CAD build for the part. Positions are in the model's coordinates, mm. Coordinates: 2 decimals unless noted, no trailing zeros. Write each loop counter-clockwise with the first axis right and the second up, starting at its lowest first coordinate (ties: lowest second). Pieces come first, ordered by that corner, then holes. Notation, with made-up numbers: (30, -9) -> (74, -9) arc R16 cw to (74, 22) -> close; hole circle Ø9 at (20, -15). An arc over 180 degrees is marked (long way). Answer as CSV lines item,"result".
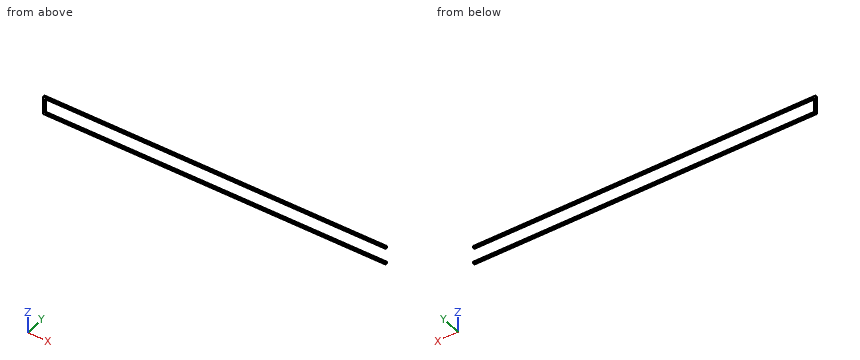
Autodesk Inventor part; units mm, degrees
ref_plane "Work Plane1" through (6.35, 0, 0) normal (1, 0, 0) x (0, 1, 0)
ref_plane "Work Plane2" through (0, 0, -6.35) normal (0, 0, 1) x (1, 0, 0)
ref_plane "XZ Plane" through (0, 0, 0) normal (0, 1, 0) x (-1, 0, 0)
sketch "Sketch1" plane through (0, 0, 0) normal (0, 1, 0) x (-1, 0, 0)
  line L0 (0, 0) -> (47.625, 0)
  line L1 (47.625, -2.54) -> (0, -2.54)
  line L2 (47.625, -2.54) -> (47.625, 0)
  dimension "d69" = 47.625
  dimension "d70" = 47.625
  dimension "d89" = 2.54
  dimension "d90" = 0
  dimension "d91" = 0
  dimension "d92" = 0
sketch "Sketch2" plane through (0, 0, 0) normal (1, 0, 0) x (0, 1, 0)
  line L0 (0, 0) -> (0.254, 0)
  line L1 (0.254, 0) -> (0.254, -0.254)
  line L2 (0.254, -0.254) -> (0, -0.254)
  line L3 (0, -0.254) -> (0, 0)
  dimension "d98" = 0.254
  dimension "d99" = 0.254
sweep "Sweep1" add profiles "Sketch2" path "Sketch1"
ref_plane "Work Plane1" through (6.35, 0, 0) normal (1, 0, 0) x (0, 1, 0)
ref_plane "Work Plane2" through (0, 0, -6.35) normal (0, 0, 1) x (1, 0, 0)
ref_plane "Work Plane4" through (0, 0, -2.9845) normal (0, 0, 1) x (1, 0, 0)
properties part number "abs_2p27" material "Silver"
Item 1: Saw through at B-B on y = 0.15. Give the cut face in (x, z) (3 decimals), and give its area (3 significant figures).
Answer below:
outline,"(-47.625, -2.54) -> (0, -2.54) -> (0, -2.286) -> (-47.371, -2.286) -> (-47.371, -0.254) -> (0, -0.254) -> (0, 0) -> (-47.625, 0) -> close"
area,"24.7 mm2"
Item 2: Wall check: line 1 (Z direction, x = -38.5, y = 0.15); line 2 (X direction, y = 0.2, z = -0.85) (3 decimals). Give the ranges that are in metal, low to high. Write a range as from..to.
Answer below:
line 1,"z = -2.54..-2.29, -0.25..0"
line 2,"x = -47.625..-47.371"
Item 3: Saw through at A-A on x = -22.5. Give the cut face in (y, z), and give its area (3 significant figures).
Answer below:
outline,"(0, -2.54) -> (0.25, -2.54) -> (0.25, -2.29) -> (0, -2.29) -> close; (0, -0.25) -> (0.25, -0.25) -> (0.25, 0) -> (0, 0) -> close"
area,"0.129 mm2"
Item 4: Saw through at C-C on z = -1.2. Give the cut face in (x, y) (3 decimals).
Answer below:
outline,"(-47.625, 0) -> (-47.371, 0) -> (-47.371, 0.254) -> (-47.625, 0.254) -> close"
